Part model, mm, in its own coordinate system. A direction names the side the tool comes from. Round coordinates to 2 decimals unless told otherwise and drop trailing zeros. Write each loop counter-clockwise with the first axis right and the second up, starting at its lowest first coordinate (ties: lowest second). Pieces come first, ordered by that corner, then holes. Notation, with made-up numbers: M -26,56.25 L 19,56.25 A28 ccw 19,84.25 Z; hole C 40,59 d11. An arc over 180 degrees is marked long. Use a Markdown table: item, result. Add a question column.
1) Drop flat-ended pins along their axis: P1, Ø3, axis at x = 1, z = 180, coming from the +Y side; P2, Ø5, axis at x = 10, y = 10, coming from the +Z side. Give the stop position or say it passes through.
2) Slice it at A-A on z = 58. Write the cut outline in (x, y).
3) Two-plate mould, pull along Y, no slides. Class faces 5 (the face through (-9, -15, 246)), 6 (the face through (3.15, 10, 246)), 7 (the face through (10, 3.15, 246)): released by +Y, released by -Y, zero draft, split by the parting line, or undercut.
4) Which spindle directions (+Z, -Z, +X, -X, +Y, -Y) get a long thin tool onto all of the face, cutting with end or side? Do faces 1 (the face through (3.15, -10, 246)), 2 (the face through (10, -3.15, 246)), 3 (the face through (-3.15, 10, 246)), 4 (the face through (-10, -3.15, 246)). Say none if no direction does.
5) Wall check: probe 1 along Y at (x, z) = (10, 273); probe 2 along X at (y, z) = (-9.25, 203.5); probe 3 along Y at (x, z) = (0, 241.5). Give the ranges that are in metal, low to high.
Autodesk Inventor part; units mm, degrees
ref_plane "YZ Plane" through (0, 0, 0) normal (1, 0, 0) x (0, 1, 0)
ref_plane "XZ Plane" through (0, 0, 0) normal (0, 1, 0) x (-1, 0, 0)
ref_plane "XY Plane" through (0, 0, 0) normal (0, 0, 1) x (1, 0, 0)
sketch "스케치1" plane through (0, 0, 0) normal (0, 0, 1) x (1, 0, 0)
  line L0 (15, 15) -> (-15, 15)
  line L1 (-15, 15) -> (-15, -15)
  line L2 (-15, -15) -> (15, -15)
  line L3 (15, -15) -> (15, 15)
  circle A0 centre (0, 0) radius 2.5
  circle A1 centre (-10, 10) radius 3
  circle A2 centre (10, 10) radius 3
  circle A3 centre (10, -10) radius 3
  circle A4 centre (-10, -10) radius 3
  line L4 (3.15, 15) -> (-3.15, 15)
  line L5 (-3.15, 15) -> (-3.15, 5)
  line L6 (-3.15, 5) -> (3.15, 5)
  line L7 (3.15, 5) -> (3.15, 15)
  line L8 (-15, -3.15) -> (-5, -3.15)
  line L9 (-5, 3.15) -> (-15, 3.15)
  line L10 (-5, -3.15) -> (-5, 3.15)
  line L11 (-15, 3.15) -> (-15, -3.15)
  line L12 (3.15, -15) -> (3.15, -5)
  line L13 (-3.15, -5) -> (-3.15, -15)
  line L14 (3.15, -5) -> (-3.15, -5)
  line L15 (-3.15, -15) -> (3.15, -15)
  line L16 (15, 3.15) -> (5, 3.15)
  line L17 (5, -3.15) -> (15, -3.15)
  line L18 (5, 3.15) -> (5, -3.15)
  line L19 (15, -3.15) -> (15, 3.15)
  dimension "d0" = 30
  dimension "d1" = 15
  dimension "d2" = 30
  dimension "d3" = 15
  dimension "d4" = 20
  dimension "d5" = 10
  dimension "d6" = 20
  dimension "d7" = 10
  dimension "d8" = 20
  dimension "d9" = 20
  dimension "d10" = 10
  dimension "d11" = 10
  dimension "d12" = 6
  dimension "d13" = 6
  dimension "d14" = 6
  dimension "d15" = 6
  dimension "d16" = 5
  dimension "d17" = 0
  dimension "d18" = 6.3
  dimension "d19" = 3.15
  dimension "d20" = 10
  dimension "d23" = 360
extrude "돌출1" add sketch "스케치1" along normal blind 500 contours L3 L16 L18 L17 L2 L12 L14 L13 L1 L8 L10 L9 L0 L5 L6 L7
equation "\"TransitionRadius\" = BendRadius"
properties part number "3030500"
Entries:
| question | item | result |
|---|---|---|
| 1 | P1 | stops at y = 5 |
| 1 | P2 | passes through |
| 2 | outline | M -15,-15 L -3.15,-15 L -3.15,-5 L 3.15,-5 L 3.15,-15 L 15,-15 L 15,-3.15 L 5,-3.15 L 5,3.15 L 15,3.15 L 15,15 L 3.15,15 L 3.15,5 L -3.15,5 L -3.15,15 L -15,15 L -15,3.15 L -5,3.15 L -5,-3.15 L -15,-3.15 Z; hole C -10,-10 d6; hole C -10,10 d6; hole C 0,0 d5; hole C 10,-10 d6; hole C 10,10 d6 |
| 3 | face 5 | released by -Y |
| 3 | face 6 | zero draft |
| 3 | face 7 | undercut |
| 4 | face 1 | +Z, -Z, -Y |
| 4 | face 2 | +Z, -Z, +X |
| 4 | face 3 | +Z, -Z, +Y |
| 4 | face 4 | +Z, -Z, -X |
| 5 | probe 1 | y = -15 to -13, -7 to -3.15, 3.15 to 7, 13 to 15 |
| 5 | probe 2 | x = -15 to -12.9, -7.1 to -3.15, 3.15 to 7.1, 12.9 to 15 |
| 5 | probe 3 | y = -5 to -2.5, 2.5 to 5 |
